For this review, take the finished solid that the model builds, in its own axes (mm). A direction names the side the tool comes from. Round coordinates to 2 decimals unless told otherwise and drop trailing zeros. Loops run counter-clockwise (first coordinate to the right, second up) from the corner with the lowest first, then second, coordinate; pieces in that order, holes last.
1) Insertion check: pin 1 (7 mm diameter, centred on x = -0.75, z = 4.35, fed in from +Y); pin 2 (1 mm diameter, centred on y = 29, z = 16.5, fed in from -X); pin 3 (3 mm diameter, centred on x = -2.5, y = 31.5, fed in from +Z); pin 4 (1.5 mm diameter, centred on y = 30.5, z = 8, fed in from -X). Each pin has a flat end and moves straight along its axis. Give the tip position at first contact, or say it passes through.
2) Take a section at D-D (x = 4). State the section outline as (y, z) points, then the cut area to 3 significant figures.
3) Mouldability with a two-part tool opening along Z and no side actions: class faces 1 (the cylindrical face through (10.74, 33.51, -15.13)), 2 (the cylindrical face through (-9.79, 31.494, 22.725)), 3 (the cylindrical face through (13.47, 33.51, -18.36)), 4 (the flat face through (-12, 32.24, -1)) as pulls with the +Z half, pulls with the -Z half, needs draft (parallel to the pull), parting line crosses it, or undercut.
4) Wall thickness on L1, parallel to Z at x = -12.75, y = 34.25 (3 decimals); L2, parallel to Z at x = 8.5, y = 32.75; L3, parallel to X at y = 26.75, z = 12: over which ranges is each line inside the solid? List them lowest first.
5) Take a section at A-A (x = -2.75). State the section outline as (y, z) points, then the cut area to 3 significant figures.
6) Take a section at C-C (z = 14). State the section outline as (x, y) points.
7) Take a section at B-B (y = 31.5). State the section outline as (x, z) points.
8) Tool access review of faces 5 (the flat face through (1, 28.24, 8)), 6 (the cylindrical face through (2.83, 27.01, 3.23)): name each direction out of +Z, -Z, +X, -X, +Y, -Y from which nothing blocks a thin tool from reaching the whole face with its end or side.
Autodesk Inventor part; units mm, degrees
ref_plane "Work Plane1" through (-12.5, 0.8429, -0.9) normal (0, 0, -1) x (0, 1, 0)
ref_plane "Work Plane2" through (8.65, 0.8429, 3.9) normal (0, 0, 1) x (1, 0, 0)
ref_plane "YZ Plane" through (0, 0, 0) normal (1, 0, 0) x (0, 1, 0)
sketch "Sketch1" plane through (0, 0, 0) normal (0, 0, 1) x (1, 0, 0)
  circle A0 centre (10.25, -9.75) radius 1.1
  circle A1 centre (-10.25, -9.75) radius 1.1
  circle A2 centre (-10.25, 3.75) radius 1.1
  circle A3 centre (10.25, 3.75) radius 1.1
  circle A4 centre (9.25, -4) radius 1.5
  circle A5 centre (-9.25, -4) radius 1.5
  arc A6 (7.25, -4) -> (11.25, -4) centre (9.25, -4) ccw
  arc A7 (-11.25, -4) -> (-7.25, -4) centre (-9.25, -4) ccw
  line L0 (8.2, -12) -> (-8.2, -12)
  line L1 (12.5, 1) -> (12.5, -7.7)
  line L2 (-12.5, 12) -> (12.5, 12)
  line L3 (-12.5, -7.7) -> (-12.5, 1)
  line L4 (12.5, -12) -> (-12.5, -12)
  line L5 (-12.5, -12) -> (-12.5, 12)
  line L6 (-12.5, 12) -> (12.5, 12)
  line L7 (12.5, 12) -> (12.5, -12)
  line L8 (-9.25, -4) -> (-9.25, -3)
  line L9 (9.25, -4) -> (9.25, -3)
  line L10 (-11.25, -4) -> (-11.25, -3)
  line L11 (-7.25, -4) -> (-7.25, -3)
  line L12 (7.25, -4) -> (7.25, -3)
  line L13 (11.25, -4) -> (11.25, -3)
  arc A8 (-9.25, -5) -> (-7.7976, -4.375) centre (-9.25, -3) ccw
  arc A9 (-7.25, -3) -> (-11.25, -3) centre (-9.25, -3) ccw
  arc A10 (9.25, -5) -> (10.7024, -4.375) centre (9.25, -3) ccw
  arc A11 (11.25, -3) -> (7.25, -3) centre (9.25, -3) ccw
  point P0 (0, 0)
  dimension "d0" = 0.5
  dimension "d1" = 0.5
  dimension "d70" = 1
  dimension "d74" = 3.25
extrude "Extrusion1" add sketch "Sketch1" along normal blind 3 contours L0 L4 L5 L3 L2 L7 L1
sketch "Sketch2" plane through (-12.5, 12, 0) normal (0, 1, 0) x (1, 0, 0)
  line L0 (25, 0) -> (0, 0)
  line L1 (0, 0) -> (0, -3)
  line L2 (25, -3) -> (0, -3)
  line L3 (25, 0) -> (25, -3)
  point P0 (12.5, 0)
extrude "Extrusion2" add sketch "Sketch2" along normal blind 2
sketch "Sketch3" plane through (-12.5, 14, 0) normal (0, 1, 0) x (1, 0, 0)
  line L0 (0, 1) -> (25, 1)
  line L1 (25, 0) -> (0, 0)
  line L2 (0, -3) -> (25, -3)
  line L3 (0, -4) -> (25, -4)
  line L4 (0, 1) -> (25, 1)
  line L5 (25, 1) -> (25, -4)
  line L6 (25, -4) -> (0, -4)
  line L7 (0, -4) -> (0, 1)
  point P0 (12.5, 0)
  dimension "d6" = 1
extrude "Extrusion3" add sketch "Sketch3" along normal blind 7.5
sketch "Sketch8" plane through (-12.5, -12, 0) normal (-1, 0, 0) x (0, 0, 1)
  line L0 (4, 24) -> (3, 24)
  line L1 (3, 26) -> (4, 26)
  line L2 (3, 0) -> (3, 26)
  line L3 (0, 0) -> (0, 26)
  line L4 (-1, 26) -> (0, 26)
  line L5 (4, 24.1) -> (3, 24.1)
  line L6 (4, 24.1) -> (-1, 24.1)
  line L7 (0, 24.1) -> (-1, 24.1)
  line L8 (-1, 24.1) -> (-1, 26)
  line L9 (-1, 26) -> (0, 26)
  line L10 (0, 26) -> (0, 24.1)
  line L11 (3, 24.1) -> (4, 24.1)
  line L12 (4, 24.1) -> (4, 26)
  line L13 (4, 26) -> (3, 26)
  line L14 (3, 26) -> (3, 24.1)
  point P0 (0, 12)
  dimension "d22" = 0.1
extrude "Extrusion7" add sketch "Sketch8" against normal up to surface (25 mm away)
sketch "Sketch9" plane through (0, 0, 3) normal (0, 0, 1) x (1, 0, 0)
  circle A0 centre (10.25, -9.75) radius 1.1
  circle A1 centre (10.25, 3.75) radius 1.1
  circle A2 centre (-10.25, 3.75) radius 1.1
  circle A3 centre (-10.25, -9.75) radius 1.1
  circle A4 centre (-10.25, -9.75) radius 1
  circle A5 centre (-10.25, 3.75) radius 1
  circle A6 centre (10.25, 3.75) radius 1
  circle A7 centre (10.25, -9.75) radius 1
  point P0 (0, 0)
  dimension "d25" = 0.1
  dimension "d26" = 0.1
  dimension "d27" = 0.1
  dimension "d28" = 0.1
ref_plane "Work Plane1" through (-12.5, 0.8429, -0.9) normal (0, 0, -1) x (0, 1, 0)
extrude "Extrusion8" add sketch "Sketch9" against normal up to surface (3.9 mm away) contours A4 | A5 | A6 | A7
sketch "Sketch10" plane through (-10.25, 3.75, 3) normal (0, 0, 1) x (1, 0, 0)
  circle A0 centre (0, 0) radius 1.1
  circle A1 centre (0, -13.5) radius 1.1
  circle A2 centre (20.5, -13.5) radius 1.1
  circle A3 centre (20.5, 0) radius 1.1
  point P0 (10.25, -3.75)
extrude "Extrusion9" add sketch "Sketch10" against normal up to surface (3 mm away)
sketch "Sketch11" plane through (0, 0, 3) normal (0, 0, 1) x (1, 0, 0)
  circle A0 centre (10.25, -9.75) radius 1
  circle A1 centre (10.25, 3.75) radius 1
  circle A2 centre (-10.25, 3.75) radius 1
  circle A3 centre (-10.25, -9.75) radius 1
  point P0 (0, 0)
ref_plane "Work Plane2" through (8.65, 0.8429, 3.9) normal (0, 0, 1) x (1, 0, 0)
extrude "Extrusion10" add sketch "Sketch11" along normal up to surface (0.9 mm away)
sketch "Sketch12" plane through (-12.5, 21.5, 4) normal (0, 0, 1) x (1, 0, 0)
  line L0 (25, -9.4) -> (25, 0)
  line L1 (25, 0) -> (25, -4.7)
  line L2 (25, -4.7) -> (30, -4.7)
  line L3 (30, -4.7) -> (30, 0)
  line L4 (30, 0) -> (25, 0)
  line L5 (25, 0) -> (25, -4.7)
  line L6 (0, -9.4) -> (0, 0)
  line L7 (0, 0) -> (25, 0)
  line L8 (0, 0) -> (-5, 0)
  line L9 (-5, 0) -> (-5, -4.7)
  line L10 (-5, -4.7) -> (0, -4.7)
  line L11 (0, -4.7) -> (0, 0)
  point P0 (12.5, -21.5)
  dimension "d35" = 5
  dimension "d36" = 5
extrude "Extrusion11" add sketch "Sketch12" against normal up to surface (5 mm away)
sketch "Sketch13" plane through (-12.5, -12, 0) normal (0, -1, 0) x (1, 0, 0)
  line L0 (0, 0) -> (0, 3)
  line L1 (25, 0) -> (25, 3)
  line L2 (25.2, 0) -> (25.2, 3)
  line L3 (-0.2, 0) -> (-0.2, 3)
  line L4 (-5, 4) -> (-5, -1)
  line L5 (-5, -1) -> (0, -1)
  line L6 (-5, 4) -> (0, 4)
  line L7 (25, -1) -> (30, -1)
  line L8 (30, 4) -> (30, -1)
  line L9 (25, 4) -> (30, 4)
  line L10 (30, -1) -> (25.2, -1)
  line L11 (25.2, -1) -> (25.2, 4)
  line L12 (25.2, 4) -> (30, 4)
  line L13 (30, 4) -> (30, -1)
  line L14 (-5, -1) -> (-0.2, -1)
  line L15 (-0.2, -1) -> (-0.2, 4)
  line L16 (-0.2, 4) -> (-5, 4)
  line L17 (-5, 4) -> (-5, -1)
  line L18 (0, 0) -> (25, 0)
  line L19 (0, 0) -> (-0.2, 0)
  line L20 (0, 3) -> (-0.2, 3)
  line L21 (25, -1) -> (25, 0)
  line L22 (25, 0) -> (25.2, 0)
  line L23 (25, 3) -> (25.2, 3)
  point P0 (12.5, 0)
  point P1 (-0.2, 3)
  point P2 (-0.2, 0)
  dimension "d39" = 0.2
  dimension "d40" = 0.2
extrude "Extrusion12" add sketch "Sketch13" against normal blind 5.5 contours L19 L3 L20 L0 | L15 L5 L4 L6 L3 | L1 L23 L2 L22 | L2 L11 L9 L8 L7
sketch "Sketch14" plane through (-12.5, -6.5, 0) normal (0, 1, 0) x (1, 0, 0)
  circle A0 centre (-2.6, -1.5) radius 1.5
  circle A1 centre (27.6, -1.5) radius 1.5
  circle A2 centre (27.6, -1.5) radius 1.4
  circle A3 centre (-2.6, -1.5) radius 1.4
  point P0 (12.5, 0)
  dimension "d43" = 0.1
  dimension "d44" = 0.1
extrude "Extrusion13" cut sketch "Sketch14" against normal blind 5.5 contours A2 | A3
chamfer "Chamfer3" distance 0.2 angle 45 8 edges at (-12.7, -9.25, 4) (-17.5, -9.25, 4) (-12.7, -9.25, -1) (-17.5, -9.25, -1) (17.5, -9.25, 4) (12.7, -9.25, 4) (17.5, -9.25, -1) (12.7, -9.25, -1)
chamfer "Chamfer4" distance 3.9999 angle 45 2 edges at (-12.5, -6.5, 1.5) (12.5, -6.5, 1.5)
sketch "Sketch15" plane through (-17.5, 16.8, 4) normal (-1, 0, 0) x (0, 0, 1)
  circle A0 centre (-2.5, 2.35) radius 1.5
  circle A1 centre (-2.5, 2.35) radius 1.4
  point P0 (-4, -16.8)
  dimension "d53" = 0.1
extrude "Extrusion14" cut sketch "Sketch15" against normal blind 5.5 contours A1
sketch "Sketch16" plane through (17.5, 16.8, 4) normal (1, 0, 0) x (0, 0, -1)
  circle A0 centre (2.5, 2.35) radius 1.4
  point P0 (4, -16.8)
extrude "Extrusion15" cut sketch "Sketch16" against normal blind 5.5
sketch "Sketch17" plane through (-12.5, 12.1, 4) normal (0, 0, 1) x (1, 0, 0)
  line L0 (25, 0) -> (25, 4.7)
  line L1 (0, 0) -> (0, 4.7)
  line L2 (30, 9.4) -> (-5, 9.4)
  line L3 (24.5905, 22.6402) -> (-1.0328, 22.6402)
  line L4 (25, 9.4) -> (0, 9.4)
  line L5 (0, 9.4) -> (0, 22.6402)
  line L6 (0, 22.6402) -> (25, 22.6402)
  line L7 (25, 22.6402) -> (25, 9.4)
  point P0 (12.5, -12.1)
  dimension "d58" = 25
extrude "Extrusion16" add sketch "Sketch17" against normal up to surface (5 mm away)
sketch "Sketch18" plane through (-12.5, 34.7402, 4) normal (0, 1, 0) x (1, 0, 0)
  circle A0 centre (22.5429, 20.4577) radius 1.5 construction
  circle A1 centre (22.5429, 20.4577) radius 1.5
  circle A2 centre (0.9195, 20.4343) radius 1.5
  circle A3 centre (22.5878, -21.1423) radius 1.5
  circle A4 centre (0.9645, -21.1657) radius 1.5
  line L0 (24.5905, -23.6401) -> (-1.0328, -23.6678)
  arc A5 (24.5905, -23.6401) -> (26.5884, -21.638) centre (24.5884, -21.6401) ccw
  line L1 (26.5873, -20.638) -> (26.5884, -21.638)
  arc A6 (-3.035, -21.67) -> (-1.0328, -23.6678) centre (-1.035, -21.6678) ccw
  line L2 (-3.035, -21.67) -> (-3.0361, -20.67)
  line L3 (26.5423, 20.962) -> (26.5434, 19.962)
  arc A7 (26.5423, 20.962) -> (24.5402, 22.9598) centre (24.5423, 20.9598) ccw
  line L4 (-1.0832, 22.9321) -> (24.5402, 22.9598)
  line L5 (-1.0832, 22.9321) -> (24.5402, 22.9598)
  arc A8 (-1.0832, 22.9321) -> (-3.081, 20.93) centre (-1.081, 20.9321) ccw
  line L6 (-3.08, 19.93) -> (-3.081, 20.93)
  line L7 (-3.08, 19.93) -> (-3.0361, -20.67)
  line L8 (26.5434, 19.962) -> (26.5873, -20.638)
  point P0 (12.5, 4)
extrude "Extrusion17" add sketch "Sketch18" against normal blind 2.5
sketch "Sketch22" plane through (-12.5, 32.2402, 4) normal (0, -1, 0) x (1, 0, 0)
  line L0 (40.0329, 38.7094) -> (-19.6341, 38.7094)
  line L1 (-19.6341, 38.7094) -> (-19.6341, -37.2102)
  line L2 (-19.6341, -37.2102) -> (40.0329, -37.2102)
  line L3 (40.0329, -37.2102) -> (40.0329, 38.7094)
  point P0 (12.5, -4)
extrude "Extrusion21" cut sketch "Sketch22" along normal blind 48.75
sketch "Sketch23" plane through (-12.5, 32.2402, 4) normal (0, -1, 0) x (1, 0, 0)
  circle A0 centre (0.9195, -20.4343) radius 1.5
  circle A1 centre (0.9645, 21.1657) radius 1.5
  circle A2 centre (22.5878, 21.1423) radius 1.5
  circle A3 centre (22.5429, -20.4577) radius 1.5
  circle A4 centre (0.9195, -20.4343) radius 3
  circle A5 centre (22.5429, -20.4577) radius 3
  circle A6 centre (22.5878, 21.1423) radius 3
  circle A7 centre (0.9645, 21.1657) radius 3
  circle A8 centre (0.9645, 21.1657) radius 1.5
  circle A9 centre (22.5878, 21.1423) radius 1.5
  circle A10 centre (0.9195, -20.4343) radius 1.5
  circle A11 centre (22.5429, -20.4577) radius 1.5
  line L0 (-3.035, 21.67) -> (-3.081, -20.93)
  arc A12 (-3.081, -20.93) -> (-1.0832, -22.9321) centre (-1.081, -20.9321) ccw
  line L1 (-1.0832, -22.9321) -> (24.5402, -22.9598)
  arc A13 (24.5402, -22.9598) -> (26.5423, -20.962) centre (24.5423, -20.9598) ccw
  line L2 (26.5423, -20.962) -> (26.5884, 21.638)
  arc A14 (26.5884, 21.638) -> (24.5905, 23.6401) centre (24.5884, 21.6401) ccw
  line L3 (24.5905, 23.6401) -> (-1.0328, 23.6678)
  arc A15 (-1.0328, 23.6678) -> (-3.035, 21.67) centre (-1.035, 21.6678) ccw
  line L4 (0.9645, 21.1657) -> (22.5429, -20.4577)
  circle A16 centre (11.7537, 0.354) radius 3.75
  line L5 (0.9645, 21.1657) -> (0.9195, -20.4343)
  line L6 (0.9195, -20.4343) -> (22.5429, -20.4577)
  line L7 (22.5878, 21.1423) -> (22.5429, -20.4577)
  line L8 (22.5878, 21.1423) -> (0.9645, 21.1657)
  point P0 (12.5, -4)
  point P1 (22.5461, -17.4577)
  point P2 (22.5846, 18.1423)
  point P3 (19.5878, 21.1455)
  point P4 (3.9645, 21.1624)
  point P5 (0.9612, 18.1657)
  point P6 (0.9227, -17.4343)
  point P7 (3.9195, -20.4375)
  point P8 (19.5429, -20.4544)
  dimension "d84" = 6
  dimension "d85" = 6
  dimension "d86" = 6
  dimension "d87" = 6
  dimension "d88" = 7.5
extrude "Extrusion22" add sketch "Sketch23" along normal blind 6.5 contours A4 L5 A7 L4 A16 A5 L6 | L4 A16 A7 L8 A6 L7 A5
sketch "Sketch26" plane through (-15.535, 34.7402, 25.67) normal (0, 1, 0) x (0.9999994, 0, -0.0010805)
  circle A0 centre (14.8117, 21.3) radius 3.75
  point P0 (15.5627, 25.6532)
extrude "Extrusion24" cut sketch "Sketch26" against normal through all
sketch "Sketch27" plane through (-15.535, 34.7402, 25.67) normal (0, 1, 0) x (0.9999994, 0, -0.0010805)
  circle A0 centre (14.8117, 21.3) radius 3.75
  circle A1 centre (14.8117, 21.3) radius 8.25
  point P0 (15.5627, 25.6532)
  dimension "d96" = 16.5
extrude "Extrusion25" cut sketch "Sketch27" against normal blind 6.5
sketch "Sketch28" plane through (10.0846, 25.7402, 22.1423) normal (0.9999994, 0, -0.0010805) x (-0.0010805, 0, -0.9999994)
  line L0 (35.6, 6.5) -> (35.6, 0)
  line L1 (35.6, 0) -> (0, 0)
  line L2 (38.6, 6.5) -> (38.6, 0)
  line L3 (38.6, 0) -> (35.6, 0)
  line L4 (39.1, 6.5) -> (-3.5, 6.5)
  line L5 (0, 6.5) -> (0, 0)
  line L6 (0, 0) -> (-3, 0)
  line L7 (-3, 6.5) -> (-3, 0)
  line L8 (28.6076, 0) -> (33.2318, -2.9777)
  line L9 (2.3601, -2.9777) -> (6.9843, 0)
  line L10 (28.6076, 0) -> (38.6, 6.5)
  line L11 (6.9843, 0) -> (-3, 6.5)
  point P0 (22.1532, -25.7402)
extrude "Extrusion26" cut sketch "Sketch28" against normal through all contours L10 L2 L3 L0 | L0 L1 L10 | L11 L5 L6 L7 | L11 L1 L5
properties part number "cameraholder_3DPrint"
Response:
1. pin 1: passes through
1. pin 2: stops at x = -11.55
1. pin 3: stops at z = 27.66
1. pin 4: stops at x = -11.55
2. outline: (25.74, -6.46) - (32.24, -16.45) - (32.24, -18.95) - (34.74, -18.95) - (34.74, -2.39) - (28.24, -2.39) - (28.24, 11.1) - (34.74, 11.1) - (34.74, 27.65) - (32.24, 27.65) - (32.24, 25.15) - (25.74, 15.16) - close
2. area: 234 mm2
3. face 1: undercut
3. face 2: pulls with the +Z half
3. face 3: pulls with the -Z half
3. face 4: needs draft
4. L1: z = -18.933 to -17.374, -15.495 to 24.285, 26.046 to 27.667
4. L2: z = -18.96 to 27.64
4. L3: x = -11.55 to 10.07
5. outline: (25.74, -6.45) - (32.24, -16.44) - (32.24, -18.94) - (34.74, -18.94) - (34.74, -3.65) - (28.24, -3.65) - (28.24, 1.18) - (25.74, 1.18) - close; (25.74, 7.52) - (28.24, 7.52) - (28.24, 12.36) - (34.74, 12.36) - (34.74, 27.66) - (32.24, 27.66) - (32.24, 25.16) - (25.74, 15.17) - close
5. area: 202 mm2
6. outline: (-15.55, 32.24) - (-11.55, 32.24) - (-11.55, 25.74) - (10.08, 25.74) - (10.08, 32.24) - (14.08, 32.24) - (14.08, 34.74) - (-15.55, 34.74) - close
7. outline: (-11.58, -13.43) arc R3 cw to (-8.8, -15.3) - (7.27, -15.32) arc R3 cw to (10.05, -13.46) - (10.08, 22.14) arc R3 cw to (7.31, 24.01) - (-8.76, 24.03) arc R3 cw to (-11.54, 22.17) - close; hole circle Ø16.5 at (-0.75, 4.35)
8. face 5: +Y
8. face 6: +Y, -Y
